Geometry check sheet. Reference: the model listing, model coordinates, mm. A direction names the side the tool comes from. Give positions to 0.01 mm unless a question says otherwise; leave off trailing zeros. Loops run counter-clockwise (first coordinate to the right, second up) from the corner with the lowest first, then second, coordinate; pieces in that order, holes last. Notation, with made-up numbers: (57.25, -2) - (110.25, -2) arc R33 ccw to (110.25, 29) - close; hole circle Ø4 at (-13, 66.5). An arc over 180 degrees is marked (long way). Use a Markdown table: item, result. Add a question column.
1. Depth check by flat-ended pin: P1, Ø6, axis at x = -18.5, y = 9.5, coming from the +Z side; P2, Ø23.5, axis at x = -0.5, y = 8, coming from the +Z side; P3, Ø12, axis at y = 12.5, z = 22.5, coming from the -X side; P4, Ø10, axis at x = -19, z = 19.5, coming from the -Y side. Enter the tip coordinate at first touch or a pass-through.
2. Cross-section at C-C on x = -6.5. Enter the section's corners in (y, z), and give its area (3 significant figures).
3. Set-up check for faces 1 (the flat face through (8.89, 22, 16)), 2 (the cylindrical face through (-21.37, 6.98, 22.27)), 3 (the flat face through (11.35, 20.51, 22.27)): record each of +Z, -Z, +X, -X, +Y, -Y from which the full face is reachable in a straight line by a thin tool's end or side.
4. Draft check along Y on faces 4 (the flat face through (-21.13, 11.97, 22.27)), 5 (the flat face through (0, 0, 0)), 6 (the cylindrical face through (11.721, -22.534, 12.522)), 7 (the flat face through (-6.48, -15.64, 22.27)). Enter one of: pulls with the +Y half, pulls with the -Y half, needs draft (parallel to the pull), parting line crosses it, or undercut.
5. Cross-section at B-B on y = 8. Enter the section's corners in (x, z), and give its area (3 significant figures).
6. Cross-section at A-A on z = 20.5. Enter the section's corners in (x, y) (3 decimals), and give its area (3 significant figures).
7. Cross-section at D-D on z = 2.5. Enter the section's corners in (x, y), and give its area (3 significant figures).
8. Material ranges on L1, parallel to Z at x = 8.5, y = -14.5; L2, parallel to Y at x = 0, z = 12.75; L3, parallel to Y at x = 12, z = 8.5, recorded low to high.
from build123d import *

# Parameters (mm, degrees)
F0_R      = 25.4
F1_DEPTH  = 25.4
F2_R      = 14.605
F3_DEPTH  = 19.05
F4_W      = 7.62
F4_H      = 3.81
F5_DEPTH  = 25.401
F8_DEPTH  = 6.35
F9_W      = 17.78
F9_H      = 6.827337
F10_DEPTH = 19.05
F12_DEPTH = 6.35


with BuildPart() as f1:
    # F0 (on Top) → F1 (new body)
    with BuildSketch(Plane.XY):
        Circle(F0_R)
    extrude(amount=F1_DEPTH)

    # F2 (on face) → F3 (cut)
    with BuildSketch(Plane.XY.offset(25.4)):
        with Locations((0, 8.255)):
            Circle(F2_R)
    extrude(amount=-F3_DEPTH, mode=Mode.SUBTRACT)

    # F4 (on Front) → F5 (cut, through all)
    with BuildSketch(Plane.XZ):
        with Locations((0, 23.495)):
            Rectangle(F4_W, F4_H)
    extrude(amount=-F5_DEPTH, mode=Mode.SUBTRACT)

    # F7 (on face) → F8 (cut)
    with BuildSketch(Plane.XY.offset(25.4)):
        Polygon((17.960513, 27.120372), (0, 9.159861), (-17.960512, 27.120374), (-27.120373, 17.960513), (-9.159862, 0), (-27.120374, -17.960511), (-17.960513, -27.120372), (0, -9.159861), (17.960512, -27.120374), (27.120373, -17.960513), (9.159862, 0), (27.120374, 17.960511), align=None)
    extrude(amount=-F8_DEPTH, mode=Mode.SUBTRACT)

    # F9 (on face) → F10 (cut, through all)
    with BuildSketch(Plane.XY.offset(25.4)):
        with Locations((0, 23.256331)):
            Rectangle(F9_W, F9_H)
    extrude(amount=-F10_DEPTH, mode=Mode.SUBTRACT)

    # F11 (on face) → F12 (cut, through all)
    with BuildSketch(Plane.XY.offset(25.4)):
        with BuildLine():
            Line((17.78, 12.065), (-17.78, 12.065))
            ThreePointArc((-17.78, 12.065), (-21.59, 8.255), (-17.78, 4.445))
            Line((-17.78, 4.445), (17.78, 4.445))
            ThreePointArc((17.78, 4.445), (21.59, 8.255), (17.78, 12.065))
        make_face()
    extrude(amount=-F12_DEPTH, mode=Mode.SUBTRACT)


solid = f1.part
Values found:
| question | item | result |
|---|---|---|
| 1 | P1 | stops at z = 25.4 |
| 1 | P2 | stops at z = 6.35 |
| 1 | P3 | stops at x = -24.55 |
| 1 | P4 | stops at y = -21.18 |
| 2 | outline | (-24.55, 0) - (24.55, 0) - (24.55, 6.35) - (-4.82, 6.35) - (-4.82, 19.05) - (-15.66, 19.05) - (-15.66, 25.4) - (-24.55, 25.4) - close |
| 2 | area | 619 mm2 |
| 3 | face 1 | +Z, +Y |
| 3 | face 2 | +Z |
| 3 | face 3 | +Z, +X |
| 4 | face 4 | pulls with the +Y half |
| 4 | face 5 | needs draft |
| 4 | face 6 | parting line crosses it |
| 4 | face 7 | undercut |
| 5 | outline | (-24.11, 0) - (24.11, 0) - (24.11, 25.4) - (21.58, 25.4) - (21.58, 19.05) - (14.6, 19.05) - (14.6, 6.35) - (-14.6, 6.35) - (-14.6, 19.05) - (-21.58, 19.05) - (-21.58, 25.4) - (-24.11, 25.4) - close |
| 5 | area | 580 mm2 |
| 6 | outline | (-21.947, -12.787) - (-10.77, -1.61) arc R14.605 cw to (-14.099, 4.445) - (-17.78, 4.445) arc R3.81 cw to (-20.285, 11.125) - (-21.947, 12.787) arc R25.4 ccw to start; (-12.787, -21.947) arc R25.4 ccw to (12.787, -21.947) - (0, -9.16) - close; (-12.787, 21.947) - (-9.865, 19.025) arc R14.605 cw to (-8.89, 19.843) - (-8.89, 23.793) arc R25.4 ccw to start; (8.89, 19.843) arc R14.605 cw to (9.865, 19.025) - (12.787, 21.947) arc R25.4 ccw to (8.89, 23.793) - close; (10.77, -1.61) - (21.947, -12.787) arc R25.4 ccw to (21.947, 12.787) - (20.285, 11.125) arc R3.81 cw to (17.78, 4.445) - (14.099, 4.445) arc R14.605 cw to start |
| 6 | area | 616 mm2 |
| 7 | outline | circle Ø50.8 at (0, 0) |
| 7 | area | 2,030 mm2 |
| 8 | L1 | z = 0 to 19.05 |
| 8 | L2 | y = -25.4 to -6.35 |
| 8 | L3 | y = -22.39 to -0.07, 16.58 to 22.39 |
